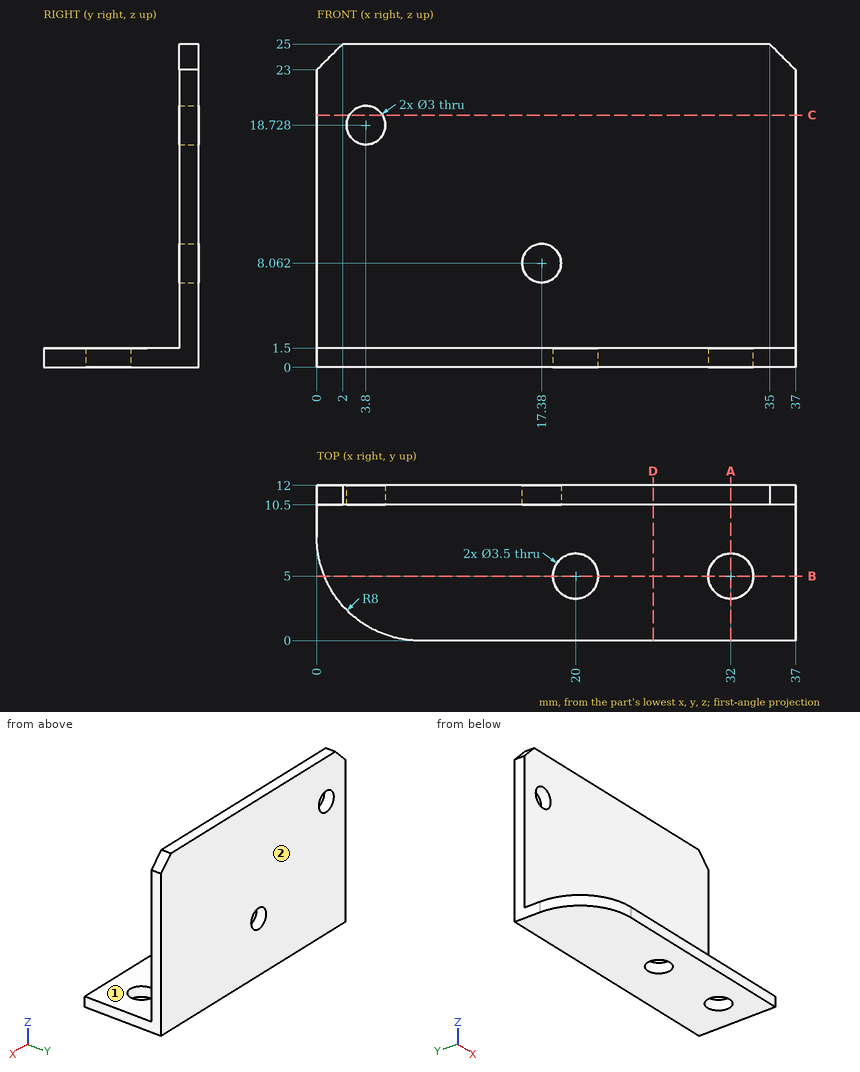
Answer from the drawing. Dimensions are ordinates in mm from the lowest x, y and z of the part. A direction names the side the tool comes from. Coordinates: 2 decimals unless noted, no trailing zeros. Write each loop counter-clockwise with the first axis right and the second up, starting at its lowest first coordinate (ties: lowest second). Pieces come first, ordered by that corner, then holes. Notation, with made-up numbers: M 4.25,-24 L 17.25,-24 A20 ccw 17.25,-18 Z; hole C 89.5,60.25 d5. An arc over 180 degrees is marked long. Put each result on its own line as item: value. Start each with the question number.
1. A cutting plane is placed at C-C on z = 19.5. Write down the section's boundary in (x, y).
2. A cutting plane is placed at B-B on y = 5. Write down the section's boundary in (x, z).
3. A cutting plane is placed at D-D on x = 26. Write down the section's boundary in (y, z).
4. A cutting plane is placed at A-A on x = 32. Write down the section's boundary in (y, z).
5. Which of the six approach directions +Z, -Z, +X, -X, +Y, -Y give full straight-line access (tool end or side, diameter ignored) to the marked faces 1 and 2?
6. Flat-ended cylindrical pins translate along their axes: P1, Ø1, axis at x = 19, z = 19, coming from the -Y side; P2, Ø5, axis at x = 32.5, y = 7, coming from the +Z side; P3, Ø6, axis at y = 2.5, z = 4, coming from the -X side. Find the tip coordinate at first contact, or state that the pin passes through.
7. Consider line 1 (Y direction, x = 20, z = 1.05); line 2 (Z direction, x = 17.38, y = 11.6); line 3 (Y direction, x = 35.5, z = 21.25). Determine where each line is inside the solid, lowest interval first. Write a range as from..to.
Resolved:
1. outline: M 0,10.5 L 2.51,10.5 L 2.51,12 L 0,12 Z; M 5.09,10.5 L 37,10.5 L 37,12 L 5.09,12 Z
2. outline: M 0.58,0 L 18.25,0 L 18.25,1.5 L 0.58,1.5 Z; M 21.75,0 L 30.25,0 L 30.25,1.5 L 21.75,1.5 Z; M 33.75,0 L 37,0 L 37,1.5 L 33.75,1.5 Z
3. outline: M 0,0 L 12,0 L 12,25 L 10.5,25 L 10.5,1.5 L 0,1.5 Z
4. outline: M 0,0 L 3.25,0 L 3.25,1.5 L 0,1.5 Z; M 6.75,0 L 12,0 L 12,25 L 10.5,25 L 10.5,1.5 L 6.75,1.5 Z
5. face 1: +Z, +X, -X, -Y
5. face 2: +Z, -Z, +X, -X, +Y
6. P1: stops at y = 10.5
6. P2: stops at z = 1.5
6. P3: stops at x = 0.98
7. line 1: y = 0..3.25, 6.75..12
7. line 2: z = 0..6.56, 9.56..25
7. line 3: y = 10.5..12
